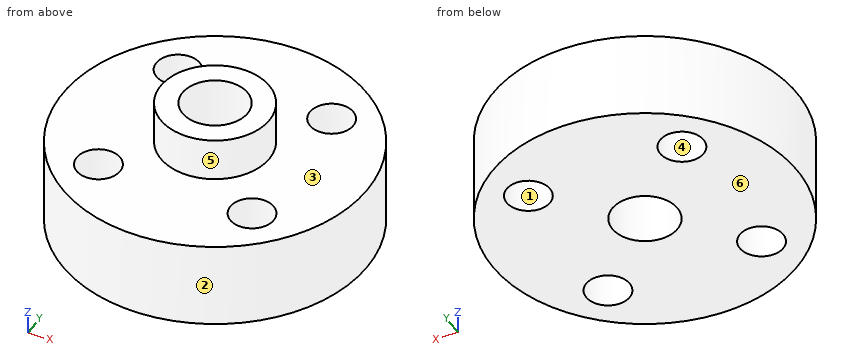
Autodesk Inventor part; units mm, degrees
ref_plane "YZ Plane" through (0, 0, 0) normal (1, 0, 0) x (0, 1, 0)
ref_plane "XZ Plane" through (0, 0, 0) normal (0, 1, 0) x (-1, 0, 0)
ref_plane "XY Plane" through (0, 0, 0) normal (0, 0, 1) x (1, 0, 0)
sketch "Sketch1" plane through (0, 0, 0) normal (0, 0, 1) x (1, 0, 0)
  circle A0 centre (0, 0) radius 11.1125
  circle A1 centre (0, 0) radius 2.3813
  circle A2 centre (0, 7.9375) radius 1.5875
  circle A3 centre (-7.9375, 0) radius 1.5875
  circle A4 centre (0, -7.9375) radius 1.5875
  circle A5 centre (7.9375, 0) radius 1.5875
  dimension "d0" = 22.225
  dimension "d1" = 4.7625
  dimension "d2" = 3.175
  dimension "d3" = 7.9375
  dimension "d6" = 360
extrude "Extrusion1" add sketch "Sketch1" along normal blind 6.35
sketch "Sketch2" plane through (0, 0, 6.35) normal (0, 0, 1) x (1, 0, 0)
  circle A0 centre (0, 0) radius 2.3813
  circle A1 centre (0, 0) radius 11.1125
  circle A2 centre (0, 0) radius 3.9688
  circle A3 centre (0, 0) radius 2.3813
  dimension "d10" = 7.9375
extrude "Extrusion2" add sketch "Sketch2" along normal blind 3.175 contours A2
sketch "Sketch4" plane through (0, 0, 6.35) normal (0, 0, 1) x (1, 0, 0)
  circle A0 centre (0, 0) radius 3.9687
  circle A1 centre (7.9375, 0) radius 1.5875
  circle A2 centre (0, -7.9375) radius 1.5875
  circle A3 centre (-7.9375, 0) radius 1.5875
  circle A4 centre (0, 7.9375) radius 1.5875
  circle A5 centre (0, 7.9375) radius 1.5875
  circle A6 centre (-7.9375, 0) radius 1.5875
  circle A7 centre (0, -7.9375) radius 1.5875
  circle A8 centre (7.9375, 0) radius 1.5875
  dimension "d22" = 360
extrude "Extrusion3" add sketch "Sketch4" against normal blind 6.35 contours A1 | A2 | A3 | A4
sketch "Sketch5" plane through (0, 0, 6.35) normal (0, 0, 1) x (1, 0, 0)
  circle A0 centre (0, 0) radius 3.9687
  circle A1 centre (0, 7.9375) radius 1.5875
  dimension "d26" = 3.175
  dimension "d27" = 7.9375
hole "Hole2" at (0, 7.9375, 6.35) direction (0, 0, -1) diameter 3.175 end through all
pattern_circular "Circular Pattern1" count 8 over 360 about axis through (0, 0, 0) along (0, 0, 1) of "Hole2"
sketch "Sketch6" plane through (0, 0, 6.35) normal (0, 0, 1) x (1, 0, 0)
  circle A0 centre (7.9375, 0) radius 1.5875
  circle A1 centre (0, -7.9375) radius 1.5875
  circle A2 centre (-7.9375, 0) radius 1.5875
  circle A3 centre (0, 7.9375) radius 1.5875
  circle A4 centre (0, 0) radius 3.9687
  circle A5 centre (0, 7.9375) radius 1.5875
  circle A6 centre (-7.9375, 0) radius 1.5875
  circle A7 centre (0, -7.9375) radius 1.5875
  circle A8 centre (7.9375, 0) radius 1.5875
  dimension "d40" = 360
extrude "Extrusion4" add sketch "Sketch6" against normal blind 6.35 contours A0 | A1 | A2 | A3
properties part number "axle hub"
Geometry check sheet. Reference: the model listing, model coordinates, mm. Face numbers are marked on the shaded views. A direction names the side the tool comes from. Give positions to 0.01 mm unless a question says otherwise; leave off trailing zeros. Loops run counter-clockwise (first coordinate to the right, second up) from the corner with the lowest first, then second, coordinate; pieces in that order, holes last. Notation, with made-up numbers: (30.5, 65) -> (39.5, 65) arc R25 cw to (39.5, 80) -> close; hole circle Ø9 at (1.5, -1.75). An arc over 180 degrees is marked (long way). Answer in a Markdown table with one row per item. Add a question column.
1) Cross-section at D-D on y = -6.75. Record the boundary of the cut face in (x, z), and give its area (3 significant figures).
2) Material ranges on probe 1 along Z at (x, y) = (3.25, -9); probe 2 along Y at (x, z) = (0, 5.75); probe 3 along X at (y, z) = (4.5, 3.75), recorded low to high. Write a range as from..to.
3) Set-up check for the marked faces 5 and 6: record each of +Z, -Z, +X, -X, +Y, -Y from which the full face is reachable in a straight line by a thin tool's end or side.
4) Draft check along X on the marked faces 1, 2, 3 and 4. Enter one of: pulls with the +X half, pulls with the -X half, needs draft (parallel to the pull), parting line crosses it, or undercut.
5) Cross-section at C-C on x = 6. Record the boundary of the cut face in (y, z), and give its area (3 significant figures).
6) Gauge pin test, flat ends, axial feed: P1, Ø4, axis at x = 4.5, z = 1.5, coming from the +Y side; P2, Ø5, axis at y = 4.5, z = 8, coming from the +X side; P3, Ø5, axis at x = 7.5, z = 3, coming from the +Y side. Record the tip position at first contact, or that the pin passes through.
Outcome:
| question | item | result |
|---|---|---|
| 1 | outline | (-8.83, 0) -> (-6.72, 0) -> (-6.72, 6.35) -> (-8.83, 6.35) -> close; (-4.51, 0) -> (4.51, 0) -> (4.51, 6.35) -> (-4.51, 6.35) -> close; (6.72, 0) -> (8.83, 0) -> (8.83, 6.35) -> (6.72, 6.35) -> close |
| 1 | area | 84.0 mm^2 |
| 2 | probe 1 | z = 0..6.35 |
| 2 | probe 2 | y = -11.11..-2.38, 2.38..11.11 |
| 2 | probe 3 | x = -10.16..-6.74, -4.48..4.48, 6.74..10.16 |
| 3 | face 5 | +Z |
| 3 | face 6 | -Z, +X, -X, +Y, -Y |
| 4 | face 1 | undercut |
| 4 | face 2 | parting line crosses it |
| 4 | face 3 | needs draft |
| 4 | face 4 | undercut |
| 5 | outline | (-9.35, 0) -> (-7.15, 0) -> (-7.15, 6.35) -> (-9.35, 6.35) -> close; (-4.07, 0) -> (4.07, 0) -> (4.07, 6.35) -> (-4.07, 6.35) -> close; (7.15, 0) -> (9.35, 0) -> (9.35, 6.35) -> (7.15, 6.35) -> close |
| 5 | area | 79.7 mm^2 |
| 6 | P1 | stops at y = 10.83 |
| 6 | P2 | stops at x = 10.8 |
| 6 | P3 | stops at y = 9.92 |
